from build123d import *

# Parameters (mm, degrees)
SKETCH_3_R          = 1.65
EXTRUDE_6_DEPTH     = 3
SKETCH_4_R          = 1
CUT_EXTRUDE_1_DEPTH = 50.497474683
FILLET_1_R          = 1


with BuildPart() as part:
    # 草图3 → 凸台-拉伸6 (new body)
    with BuildSketch(Plane(origin=(0, 0, 0), x_dir=(1, 0, 0), z_dir=(0, 1, 0))):
        Polygon((-37, -20.5), (-40, -20.5), (-40, -8.5), (-37, -8.5), (-37, 0), (37, 0), (37, -8.5), (40, -8.5), (40, -20.5), (37, -20.5), (37, -29), (-37, -29), align=None)
        with Locations(Location((-10, -2.3, 0), (0, 0, 270))):
            Circle(SKETCH_3_R, mode=Mode.SUBTRACT)
        with Locations(Location((10, -2.3, 0), (0, 0, 270))):
            Circle(SKETCH_3_R, mode=Mode.SUBTRACT)
        with Locations(Location((0, -26, 0), (0, 0, 270))):
            Circle(SKETCH_3_R, mode=Mode.SUBTRACT)
        with Locations(Location((-21.5, -14.15, 0), (0, 0, 270))):
            Circle(SKETCH_3_R, mode=Mode.SUBTRACT)
        with Locations(Location((21.5, -14.15, 0), (0, 0, 90))):
            Circle(SKETCH_3_R, mode=Mode.SUBTRACT)
    extrude(amount=EXTRUDE_6_DEPTH)

    # 草图4 → 切除-拉伸1 (cut, through all)
    with BuildSketch(Plane(origin=(0, 3, 0), x_dir=(1, 0, 0), z_dir=(0, 1, 0))):
        with Locations((-37, -7.5)):
            Circle(SKETCH_4_R)
        with Locations((-37, -21.5)):
            Circle(SKETCH_4_R)
        with Locations((37, -21.5)):
            Circle(SKETCH_4_R)
        with Locations((37, -7.5)):
            Circle(SKETCH_4_R)
        with BuildLine():
            Line((-33, -4), (-17.977516568, -4))
            Line((-17.977516568, -4), (-22.460716028, -10.267085539))
            ThreePointArc((-22.460716028, -10.267085539), (-24.753285657, -11.822741434), (-25.485103536, -14.494891011))
            Line((-25.485103536, -14.494891011), (-33, -25))
            Line((-33, -25), (-33, -4))
        make_face()
        with BuildLine():
            Line((-28.08189514, -25), (-22.978936608, -17.866550351))
            ThreePointArc((-22.978936608, -17.866550351), (-18.246714343, -16.477258566), (-18.460311642, -11.549943331))
            Line((-18.460311642, -11.549943331), (-13.059411708, -4))
            ThreePointArc((-13.059411708, -4), (-12.079761561, -5.115065159), (-10.726079501, -5.723858723))
            Line((-10.726079501, -5.723858723), (-2.959290121, -24.131149556))
            ThreePointArc((-2.959290121, -24.131149556), (-3.186448679, -24.552054968), (-3.354101966, -25))
            Line((-3.354101966, -25), (-28.08189514, -25))
        make_face()
        Polygon((-7.111954792, -4), (7.111954792, -4), (0, -20.855332858), align=None)
        with BuildLine():
            Line((33, -25), (33, -4))
            Line((33, -4), (17.977516568, -4))
            Line((17.977516568, -4), (22.460716028, -10.267085539))
            ThreePointArc((22.460716028, -10.267085539), (24.753285657, -11.822741434), (25.485103536, -14.494891011))
            Line((25.485103536, -14.494891011), (33, -25))
        make_face()
        with BuildLine():
            Line((3.354101966, -25), (28.08189514, -25))
            Line((28.08189514, -25), (22.978936608, -17.866550351))
            ThreePointArc((22.978936608, -17.866550351), (18.246714343, -16.477258566), (18.460311642, -11.549943331))
            Line((18.460311642, -11.549943331), (13.059411708, -4))
            ThreePointArc((13.059411708, -4), (12.079761561, -5.115065159), (10.726079501, -5.723858723))
            Line((10.726079501, -5.723858723), (2.959290121, -24.131149556))
            ThreePointArc((2.959290121, -24.131149556), (3.186448679, -24.552054968), (3.354101966, -25))
        make_face()
    extrude(amount=-CUT_EXTRUDE_1_DEPTH, mode=Mode.SUBTRACT)

    # 圆角1
    # the kernel refuses this fillet: 1 mm, written as the material it adds along each edge
    with BuildSketch(Plane(origin=(17.977516568, 3, 4), x_dir=(1, 0, 0), z_dir=(0, -1, 0)), Plane(origin=(-28.08189514, 3, 25), x_dir=(0.5818146414920115, 0, -0.8133214142917436), z_dir=(0, -1, 0)), Plane(origin=(-17.977516568, 3, 4), x_dir=(-0.5818146414920105, 0, 0.8133214142917444), z_dir=(0, -1, 0))) as fillet_1_piece_1:
        with BuildLine():
            CenterArc((FILLET_1_R * 1.94488256881, FILLET_1_R), FILLET_1_R, 144.421723672, 125.578276328)
            Line((FILLET_1_R * 1.13156115451, FILLET_1_R * 1.58181464149), (0, 0))
            Line((0, 0), (FILLET_1_R * 1.94488256881, 0))
        make_face()
    extrude(amount=3)
    with BuildSketch(Plane(origin=(33, 3, 4), x_dir=(-1, 0, 0), z_dir=(0, -1, 0)), Plane(origin=(-33, 3, 4), x_dir=(0, 0, 1), z_dir=(0, -1, 0))) as fillet_1_piece_2:
        with BuildLine():
            CenterArc((FILLET_1_R, -FILLET_1_R), FILLET_1_R, 90, 90)
            Line((0, -FILLET_1_R), (0, 0))
            Line((0, 0), (FILLET_1_R, 0))
        make_face()
    extrude(amount=3)
    with BuildSketch(Plane(origin=(2.959290121, 3, 24.131149556), x_dir=(0.38875206983693955, 0, -0.9213424055135502), z_dir=(0, -1, 0))) as fillet_1_piece_3:
        with BuildLine():
            CenterArc((0.481820643, 1), FILLET_1_R, 221.810314896, 48.189685104)
            ThreePointArc((-0.26353535, 0.333333333), (-0.126704365, 0.17066975), (0, 0))
            Line((0, 0), (0.481820643, 0))
        make_face()
    extrude(amount=3)
    with BuildSketch(Plane(origin=(10.726079501, 3, 5.723858723), x_dir=(-0.38875206983694, 0, 0.92134240551355), z_dir=(0, -1, 0)), Plane(origin=(-2.959290121, 3, 24.131149556), x_dir=(-0.38875206983693955, 0, -0.9213424055135502), z_dir=(0, -1, 0))) as fillet_1_piece_4:
        with BuildLine():
            CenterArc((0.481820643, -1), FILLET_1_R, 90, 48.189685104)
            ThreePointArc((-0.26353535, -0.333333333), (-0.126704365, -0.17066975), (0, 0))
            Line((0, 0), (0.481820643, 0))
        make_face()
    extrude(amount=3)
    with BuildSketch(Plane(origin=(13.059411708, 3, 4), x_dir=(-0.6232784406716191, 0, 0.7819999906610966), z_dir=(0, -1, 0))) as fillet_1_piece_5:
        with BuildLine():
            CenterArc((1.319920856, -0.986295222), FILLET_1_R, 99.496659768, 96.369123068)
            Line((0.358016109, -1.259680038), (0, 0))
            ThreePointArc((0, 0), (0.577465375, -0.047966724), (1.154930749, 0))
        make_face()
    extrude(amount=3)
    with BuildSketch(Plane(origin=(18.460311642, 3, 11.549943331), x_dir=(-0.5818146414920088, 0, -0.8133214142917455), z_dir=(0, -1, 0)), Plane(origin=(-22.978936608, 3, 17.866550351), x_dir=(-0.581814641492012, 0, 0.8133214142917432), z_dir=(0, -1, 0))) as fillet_1_piece_6:
        with BuildLine():
            CenterArc((0.716825297, -1), FILLET_1_R, 90, 66.927317505)
            ThreePointArc((-0.203183154, -0.608101481), (-0.089388104, -0.308128251), (0, 0))
            Line((0, 0), (0.716825297, 0))
        make_face()
    extrude(amount=3)
    with BuildSketch(Plane(origin=(22.978936608, 3, 17.866550351), x_dir=(-0.9557806548183481, 0, 0.29408049897096183), z_dir=(0, -1, 0)), Plane(origin=(-18.460311642, 3, 11.549943331), x_dir=(0.5870204705662555, 0, 0.8095720889063382), z_dir=(0, -1, 0))) as fillet_1_piece_7:
        with BuildLine():
            CenterArc((0.721291541, -0.996783336), FILLET_1_R, 94.59681443, 66.927317505)
            Line((-0.227165673, -0.679878124), (0, 0))
            ThreePointArc((0, 0), (0.320574018, -0.012866657), (0.641148037, 0))
        make_face()
    extrude(amount=3)
    with BuildSketch(Plane(origin=(28.08189514, 3, 25), x_dir=(-0.5818146414920125, 0, -0.813321414291743), z_dir=(0, -1, 0))) as fillet_1_piece_8:
        with BuildLine():
            CenterArc((FILLET_1_R * 1.94488256881, -FILLET_1_R), FILLET_1_R, 90, 125.578276328)
            Line((FILLET_1_R * 1.13156115451, -FILLET_1_R * 1.58181464149), (0, 0))
            Line((0, 0), (FILLET_1_R * 1.94488256881, 0))
        make_face()
    extrude(amount=3)
    with BuildSketch(Plane(origin=(3.354101966, 3, 25), x_dir=(1, 0, 0), z_dir=(0, -1, 0))) as fillet_1_piece_9:
        with BuildLine():
            CenterArc((0.677026908, -1), FILLET_1_R, 90, 63.612200039)
            ThreePointArc((-0.218779509, -0.555555556), (-0.09752127, -0.282451624), (0, 0))
            Line((0, 0), (0.677026908, 0))
        make_face()
    extrude(amount=3)
    with BuildSketch(Plane(origin=(-13.059411708, 3, 4), x_dir=(-0.5818146414920109, 0, 0.8133214142917442), z_dir=(0, -1, 0))) as fillet_1_piece_10:
        with BuildLine():
            CenterArc((1.309568376, -1), FILLET_1_R, 90, 96.369123068)
            ThreePointArc((0.31574053, -1.11093337), (0.204009684, -0.542353311), (0, 0))
            Line((0, 0), (1.309568376, 0))
        make_face()
    extrude(amount=3)
    with BuildSketch(Plane(origin=(-10.726079501, 3, 5.723858723), x_dir=(-0.9638482393906854, 0, -0.26645181820260827), z_dir=(0, -1, 0))) as fillet_1_piece_11:
        with BuildLine():
            CenterArc((0.485629561, -0.99815583), FILLET_1_R, 93.480205158, 48.189685104)
            Line((-0.298820999, -0.377964473), (0, 0))
            ThreePointArc((0, 0), (0.212462933, -0.006454594), (0.424925866, 0))
        make_face()
    extrude(amount=3)
    with BuildSketch(Plane(origin=(-3.354101966, 3, 25), x_dir=(0.3664147496948947, 0, -0.9304516275476269), z_dir=(0, -1, 0))) as fillet_1_piece_12:
        with BuildLine():
            CenterArc((0.682378983, -0.996355538), FILLET_1_R, 94.893125181, 63.612200039)
            Line((-0.248072645, -0.629940788), (0, 0))
            ThreePointArc((0, 0), (0.298540805, -0.012755617), (0.59708161, 0))
        make_face()
    extrude(amount=3)
    with BuildSketch(Plane(origin=(-7.111954792, 3, 4), x_dir=(0.38875206983694144, 0, 0.9213424055135496), z_dir=(0, -1, 0))) as fillet_1_piece_13:
        with BuildLine():
            CenterArc((FILLET_1_R * 1.507313743, -FILLET_1_R), FILLET_1_R, 90, 112.876871805)
            Line((FILLET_1_R * 0.585971337484, -FILLET_1_R * 1.38875206984), (0, 0))
            Line((0, 0), (FILLET_1_R * 1.507313743, 0))
        make_face()
    extrude(amount=3)
    with BuildSketch(Plane(origin=(7.111954792, 3, 4), x_dir=(-0.38875206983694094, 0, 0.9213424055135497), z_dir=(0, -1, 0))) as fillet_1_piece_14:
        with BuildLine():
            CenterArc((FILLET_1_R * 1.507313743, FILLET_1_R), FILLET_1_R, 157.123128195, 112.876871805)
            Line((FILLET_1_R * 0.585971337484, FILLET_1_R * 1.38875206984), (0, 0))
            Line((0, 0), (FILLET_1_R * 1.507313743, 0))
        make_face()
    extrude(amount=3)
    with BuildSketch(Plane(origin=(0, 3, 20.855332858), x_dir=(0.38875206983694144, 0, -0.9213424055135495), z_dir=(0, -1, 0))) as fillet_1_piece_15:
        with BuildLine():
            CenterArc((FILLET_1_R * 2.37, -FILLET_1_R), FILLET_1_R, 90, 134.246256391)
            Line((FILLET_1_R * 1.65365246566, -FILLET_1_R * 1.69774365639), (0, 0))
            Line((0, 0), (FILLET_1_R * 2.37, 0))
        make_face()
    extrude(amount=3)
    with BuildSketch(Plane(origin=(33, 3, 25), x_dir=(0, 0, -1), z_dir=(0, -1, 0)), Plane(origin=(-33, 3, 25), x_dir=(0.5818146414920113, 0, -0.8133214142917439), z_dir=(0, -1, 0))) as fillet_1_piece_16:
        with BuildLine():
            CenterArc((FILLET_1_R * 3.11666514552, -FILLET_1_R), FILLET_1_R, 90, 144.421723672)
            Line((FILLET_1_R * 2.53485050403, -FILLET_1_R * 1.81332141429), (0, 0))
            Line((0, 0), (FILLET_1_R * 3.11666514552, 0))
        make_face()
    extrude(amount=3)
    with BuildSketch(Plane(origin=(25.485103536, 3, 14.494891011), x_dir=(0.5818146414920119, 0, 0.8133214142917433), z_dir=(0, -1, 0)), Plane(origin=(-22.460716028, 3, 10.267085539), x_dir=(0.5818146414920021, 0, -0.8133214142917503), z_dir=(0, -1, 0))) as fillet_1_piece_17:
        with BuildLine():
            CenterArc((0.346117617, -1), FILLET_1_R, 90, 36.089146464)
            ThreePointArc((-0.242925672, -0.191898519), (-0.11960566, -0.098300271), (0, 0))
            Line((0, 0), (0.346117617, 0))
        make_face()
    extrude(amount=3)
    with BuildSketch(Plane(origin=(22.460716028, 3, 10.267085539), x_dir=(0.9607072883816618, 0, 0.277563517145814), z_dir=(0, -1, 0)), Plane(origin=(-25.485103536, 3, 14.494891011), x_dir=(-0.04760515714824153, 0, -0.99886623179127), z_dir=(0, -1, 0))) as fillet_1_piece_18:
        with BuildLine():
            CenterArc((0.348274134, -0.999250986), FILLET_1_R, 92.217735732, 36.089146464)
            Line((-0.271599158, -0.214549067), (0, 0))
            ThreePointArc((0, 0), (0.154788504, -0.002996057), (0.309577008, 0))
        make_face()
    extrude(amount=3)
    # the kernel refuses this fillet: 1 mm, written as the material it takes off along each edge
    with BuildSketch(Plane(origin=(-37, -2.5, 0), x_dir=(0, 0, 1), z_dir=(0, 1, 0)), Plane(origin=(37, -2.5, 0), x_dir=(-1, 0, 0), z_dir=(0, 1, 0)), Plane(origin=(40, -2.5, 8.5), x_dir=(-1, 0, 0), z_dir=(0, 1, 0)), Plane(origin=(40, -2.5, 20.5), x_dir=(0, 0, -1), z_dir=(0, 1, 0)), Plane(origin=(37, -2.5, 29), x_dir=(0, 0, -1), z_dir=(0, 1, 0)), Plane(origin=(-40, -2.5, 20.5), x_dir=(1, 0, 0), z_dir=(0, 1, 0)), Plane(origin=(-40, -2.5, 8.5), x_dir=(0, 0, 1), z_dir=(0, 1, 0))) as fillet_1_2_piece_1:
        with BuildLine():
            CenterArc((FILLET_1_R, FILLET_1_R), FILLET_1_R, 180, 90)
            Line((0, FILLET_1_R), (0, 0))
            Line((0, 0), (FILLET_1_R, 0))
        make_face()
    extrude(amount=8, mode=Mode.SUBTRACT)
    with BuildSketch(Plane(origin=(-37, -2.5, 29), x_dir=(0, 0, -1), z_dir=(0, 1, 0))) as fillet_1_2_piece_2:
        with BuildLine():
            CenterArc((FILLET_1_R, -FILLET_1_R), FILLET_1_R, 90, 90)
            Line((0, -FILLET_1_R), (0, 0))
            Line((0, 0), (FILLET_1_R, 0))
        make_face()
    extrude(amount=8, mode=Mode.SUBTRACT)


solid = part.part
Geometry: final body of the model. Coordinates: model frame, mm. A direction names the side the tool comes from. Round coordinates to 2 decimals unless told otherwise and drop trailing zeros. Loops run counter-clockwise (first coordinate to the right, second up) from the corner with the lowest first, then second, coordinate; pieces in that order, holes last.
Q1. Section C-C on z = 26. Return loops of the section in (x, y).
Q2. Pull-direction query (X, two-part tool) for faces 1 (the flat face through (-38, 1, 8.5)), 2 (the flat face through (-37, 1, 4)), 3 (the flat face through (0, 2, 4)); classes: released by +X, released by -X, zero draft, split by the parting line, or undercut.
Q3. Section A-A on z = 2.3. Return loops of the section in (x, y), plus the area to 3 significant figures.
Q4. Access query for faces 4 (the flat face through (38, 1, 8.5)), 5 (the flat face through (1, 1, 29)), 6 (the cylindrical face through (-19.04, 1.52, 4.53)), 7 (the flat face through (37, 1, 25)). Directions: +Z, -Z, +X, -X, +Y, -Y. A direction counts if a zero-diameter tool reaches every point of the face in a straight line with its end or side. Return the directions, or none.
Q5. Section D-D on y = 2.35. State how many separate pieces and enclosed holes the cut face has, plus the area to 3 significant figures.
Q6. Material intervals for L1, parallel to X at y = 2, z = 2.3; L2, parallel to Z at x = -11, y = 2.85; L3, parallel to Z at x = 20, y = 1.6, sorted ascending.
Q7. Section B-B on x = 21.5. Return loops of the section in (y, z).
Q8. Pin query (flat end, axial travel): P1, Ø0.6, axis at x = 38.5, y = 1.5, coming from the -Z side; P2, Ø1.5, axis at y = 1.5, z = 21.5, coming from the +X side; P3, Ø1.5, axis at y = 1, z = 24.5, coming from the -X side. Return the tip coordinate at first contact, or that it passes through.
Evaluation:
1. outline: (-37, 0) - (-1.65, 0) - (-1.65, 3) - (-37, 3) - close; (1.65, 0) - (37, 0) - (37, 3) - (1.65, 3) - close
2. face 1: zero draft
2. face 2: released by -X
2. face 3: undercut
3. outline: (-37, 0) - (-11.65, 0) - (-11.65, 3) - (-37, 3) - close; (-8.35, 0) - (8.35, 0) - (8.35, 3) - (-8.35, 3) - close; (11.65, 0) - (37, 0) - (37, 3) - (11.65, 3) - close
3. area: 202 mm2
4. face 4: -Z, +X, +Y, -Y
4. face 5: +Z, +X, -X, +Y, -Y
4. face 6: +Y, -Y
4. face 7: +Z, +X, +Y, -Y
5. separate pieces: 1
5. enclosed holes: 10
5. area: 1,220 mm2
6. L1: x = -37 to -11.65, -8.35 to 8.35, 11.65 to 37
6. L2: z = 0 to 0.99, 3.61 to 5.67, 25 to 29
6. L3: z = 0 to 4, 6.83 to 13.46, 14.84 to 17.86, 25 to 29
7. outline: (0, 0) - (3, 0) - (3, 4) - (0, 4) - close; (0, 8.92) - (3, 8.92) - (3, 12.5) - (0, 12.5) - close; (0, 15.8) - (3, 15.8) - (3, 18.15) - (0, 18.15) - close; (0, 25) - (3, 25) - (3, 29) - (0, 29) - close
8. P1: stops at z = 8.5
8. P2: stops at x = 36.34
8. P3: stops at x = -37
